Could you check a few things on this model? Use its own coordinates, in mm. Face numbers are marked on the shaded views. A direction names the side the tool comes from. Round coordinates to 2 decimals unless told otherwise and drop trailing zeros. Loops run counter-clockwise (first coordinate to the right, second up) from the corner with the lowest first, then second, coordinate; pieces in that order, holes last. Notation, with made-up numbers: (43.5, 16.5) -> (73.5, 16.5) arc R20 ccw to (73.5, 48.5) -> close; hole circle Ø3 at (10.5, 36.5). An arc over 180 degrees is marked (long way). Use CSV: the item, a comma, the result in double quotes. Start each with the question number.
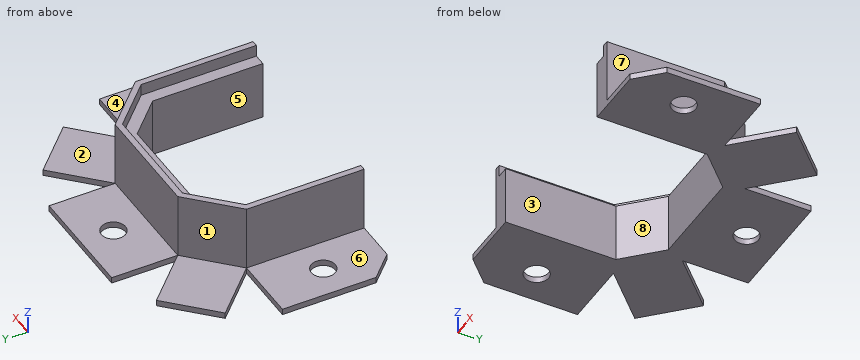
```python
from build123d import *

# Parameters (mm, degrees)
F4_D     = 12.7
F4_DEPTH = 12.7
F4_TIP   = 3.8154649308
F6_DEPTH = 3.176
F7_SIZE  = 12.7


# Not quite as in the source:
# - a feature names something its author has since deleted; it is built from what else it names


with BuildPart() as f2:
    # F2: sweep along a path in F1
    with BuildLine(Plane.XY) as f2_path:
        Line((-44.45, 0), (-44.45, 58.2394877579))
        Line((-44.45, 58.2394877579), (-26.4894877579, 76.2))
        Line((-26.4894877579, 76.2), (26.4894877579, 76.2))
        Line((26.4894877579, 76.2), (44.45, 58.2394877579))
        Line((44.45, 58.2394877579), (44.45, 0))
    # F0 (on Front) → F2 (sweep)
    with BuildSketch(Plane.XZ):
        Polygon((-50.8, 38.1), (-53.975, 38.1), (-53.975, 3.175), (-88.9, 3.175), (-88.9, 0), (-53.975, 0), (-50.8, 0), (-50.8, 3.175), (-50.8, 31.75), align=None)
        Polygon((-44.45, 31.75), (-50.8, 31.75), (-50.8, 3.175), (-50.8, 0), (-44.45, 0), align=None)
    sweep(path=f2_path.line, transition=Transition.RIGHT)

    # F4
    with Locations(Plane.XY.offset(3.175)):
        with Locations((-71.4375, 31.0896), (71.4375, 31.0896), (0, 103.1875)):
            Hole(F4_D / 2, depth=F4_DEPTH)
            with Locations((0, 0, -(F4_DEPTH + F4_TIP / 2))):  # 118° drill point
                Cone(0, F4_D / 2, F4_TIP, mode=Mode.SUBTRACT)

    # F5 (on face) → F6 (cut, through all)
    with BuildSketch(Plane.XY.offset(3.175)):
        Polygon((-88.9, 62.1848719395), (-53.975, 62.1848719395), (-78.6707043329, 86.8805762724), (-88.9, 76.6512806053), align=None)
        Polygon((-55.1305762724, 110.4207043329), (-30.4348719395, 85.725), (-30.4348719395, 120.65), (-44.9012806053, 120.65), align=None)
        Polygon((30.4348719395, 120.65), (30.4348719395, 85.725), (55.1305762724, 110.4207043329), (44.9012806053, 120.65), align=None)
        Polygon((78.6707043329, 86.8805762724), (53.975, 62.1848719395), (88.9, 62.1848719395), (88.9, 76.6512806053), align=None)
    extrude(amount=-F6_DEPTH, mode=Mode.SUBTRACT)

    # F7
    f7_edges = [f2.edges().sort_by_distance(p)[0] for p in [
        (-88.9, 0, 1.5875),
        (88.9, 0, 1.5875),
    ]]
    chamfer(f7_edges, length=F7_SIZE)


solid = f2.part
```
1. Will these pins go through, and if not, where does the flat tip stop? pin 1 (10 mm diameter, centred on x = -64.5, z = 9.5, fed in from +Y); pin 2 (5 mm diameter, centred on x = 20, z = 28, fed in from -Y); pin 3 (17.5 mm diameter, centred on x = -12.5, y = 95.5, fed in from +Z) (3 decimals); pin 4 (10.5 mm diameter, centred on x = -2.5, z = 12, fed in from +Y) (3 decimals).
2. Suppose I cut it at A-A (y = 55). List the corners of the cut face in (x, z) for me (3 decimals), then the cut area to 3 significant figures.
3. If I drill on L1, parallel to X at y = 32, z = 5.5 (3 decimals); L2, parallel to X at y = 33, z = 34 (3 decimals); L3, parallel to Y at x = 0, z = 1.1, over which ranges is the centre line in solid material (lowest first)?
4. Suppose I cut it at D-D (y = 99.5). List the corners of the cut face in (x, z) for me (3 decimals).
5. We'd pull the mould along X, two halves only. Please class the marked faces 5, 6, 7 and 8: pulls with the +X half, pulls with the -X half, needs draft (parallel to the pull), parting line crosses it, or undercut.
6. For the marked faces 1, 2, 3 and 4, which set-ups out of +Z, -Z, +X, -X, +Y, -Y let a thin tool reach every point of the face, with its end or its side?
7. Suppose I cut it at C-C (x = 20). List the corners of the cut face in (y, z) for me (3 decimals), then the cut area to 3 significant figures.
Geometry check:
1,pin 1,"passes through"
1,pin 2,"stops at y = 76.2"
1,pin 3,"stops at z = 3.175"
1,pin 4,"stops at y = 85.725"
2,outline,"(-88.9, 0) -> (-44.45, 0) -> (-44.45, 31.75) -> (-50.8, 31.75) -> (-50.8, 38.1) -> (-53.975, 38.1) -> (-53.975, 3.175) -> (-88.9, 3.175) -> close; (44.45, 0) -> (88.9, 0) -> (88.9, 3.175) -> (53.975, 3.175) -> (53.975, 38.1) -> (50.8, 38.1) -> (50.8, 31.75) -> (44.45, 31.75) -> close"
2,area,"867 mm²"
3,L1,"x = -53.975 to -44.45, 44.45 to 53.975"
3,L2,"x = -53.975 to -50.8, 50.8 to 53.975"
3,L3,"y = 76.2 to 96.84, 109.54 to 120.65"
4,outline,"(-66.051, 0) -> (-44.21, 0) -> (-44.21, 3.175) -> (-66.051, 3.175) -> close; (-30.435, 0) -> (-5.17, 0) -> (-5.17, 3.175) -> (-30.435, 3.175) -> close; (5.17, 0) -> (30.435, 0) -> (30.435, 3.175) -> (5.17, 3.175) -> close; (44.21, 0) -> (66.051, 0) -> (66.051, 3.175) -> (44.21, 3.175) -> close"
5,face 5,"undercut"
5,face 6,"needs draft"
5,face 7,"pulls with the +X half"
5,face 8,"undercut"
6,face 1,"+Z, -X, +Y"
6,face 2,"+Z, +X, +Y"
6,face 3,"+Z, -Z, -Y"
6,face 4,"+Z, +X, +Y, -Y"
7,outline,"(76.2, 0) -> (120.65, 0) -> (120.65, 3.175) -> (85.725, 3.175) -> (85.725, 38.1) -> (82.55, 38.1) -> (82.55, 31.75) -> (76.2, 31.75) -> close"
7,area,"433 mm²"
